Read the model definition and answer for the solid it produces. Units are mm, in the model's axes. A direction names the side the tool comes from. Give positions to 0.01 mm unless a question says otherwise; leave off trailing zeros. Order: outer loops, then holes, each group sorted by start corner. A loop starts at its lowest first (then second) coordinate and runs counter-clockwise, first axis right, second up. Notation, with made-up numbers: (35, 8) - (89, 8) arc R19 cw to (89, 44) - close; hole circle Ø11 at (-31.5, 11.25). An arc over 180 degrees is marked (long way). Write item = value, one per line.
```python
from build123d import *

# Parameters (mm, degrees)
SKETCH1_R                = 19.05
SKETCH1_R_2              = 12.7
BOSS_EXTRUDE1_DEPTH      = 571.5
BOSS_EXTRUDE2_START      = -12.7
SKETCH2_R                = 50.8
SKETCH2_R_2              = 12.7
BOSS_EXTRUDE2_DEPTH      = 12.7
SKETCH3_R                = 50.8
SKETCH3_R_2              = 12.7
BOSS_EXTRUDE3_DEPTH      = 12.7
BOSS_EXTRUDE4_REACH      = 609.748
BOSS_EXTRUDE4_END_RADIUS = 19.05
BOSS_EXTRUDE4_START      = 31.75
SKETCH4_W                = 25.4
SKETCH4_H                = 25.4
SKETCH4_R                = 2.286


with BuildPart() as part:
    # Sketch1 → Boss-Extrude1 (new, symmetric)
    with BuildSketch(Plane(origin=(0, 0, 0), x_dir=(0, 0, -1), z_dir=(1, 0, 0))):
        Circle(SKETCH1_R)
        Circle(SKETCH1_R_2, mode=Mode.SUBTRACT)
    extrude(amount=BOSS_EXTRUDE1_DEPTH, both=True)

    # Sketch2 → Boss-Extrude2 (add)
    with BuildSketch(Plane(origin=(571.5, 0, 0), x_dir=(0, 0, -1), z_dir=(1, 0, 0)).offset(BOSS_EXTRUDE2_START)):
        Circle(SKETCH2_R)
        Circle(SKETCH2_R_2, mode=Mode.SUBTRACT)
    extrude(amount=BOSS_EXTRUDE2_DEPTH)

    # Sketch3 → Boss-Extrude3 (add)
    with BuildSketch(Plane.ZY.offset(571.5)):
        with Locations(Location((0, 0, 0), (0, 0, 180))):
            Circle(SKETCH3_R)
        with Locations(Location((0, 0, 0), (0, 0, 180))):
            Circle(SKETCH3_R_2, mode=Mode.SUBTRACT)
    extrude(amount=-BOSS_EXTRUDE3_DEPTH)

    # Boss-Extrude4: up to this cylinder (the profile starts outside it)
    boss_extrude4_end = Plane(origin=(-6.170395, 0, 0), z_dir=(-1, 0, 0)) * Cylinder(BOSS_EXTRUDE4_END_RADIUS, 2008.25521, mode=Mode.PRIVATE)
    # Sketch4 → Boss-Extrude4 (add, up to the surface)
    with BuildSketch(Plane(origin=(0, 0, 0), x_dir=(1, 0, 0), z_dir=(0, 1, 0)).offset(BOSS_EXTRUDE4_START), mode=Mode.PRIVATE) as boss_extrude4_sk1:
        with Locations((-381, 0)):
            Rectangle(SKETCH4_W, SKETCH4_H)
        with Locations(Location((-381, 0, 0), (0, 0, 270))):
            Circle(SKETCH4_R, mode=Mode.SUBTRACT)
    boss_extrude4_tool1 = extrude(boss_extrude4_sk1.sketch, amount=-BOSS_EXTRUDE4_REACH, mode=Mode.PRIVATE) - boss_extrude4_end
    add(boss_extrude4_tool1.solids().sort_by_distance((-381, 31.75, 12.34079))[0])
    # Sketch4 → Boss-Extrude4 (add, up to the surface)
    with BuildSketch(Plane(origin=(0, 0, 0), x_dir=(1, 0, 0), z_dir=(0, 1, 0)).offset(BOSS_EXTRUDE4_START), mode=Mode.PRIVATE) as boss_extrude4_sk2:
        with Locations((381, 0)):
            Rectangle(SKETCH4_W, SKETCH4_H)
        with Locations(Location((381, 0, 0), (0, 0, 270))):
            Circle(SKETCH4_R, mode=Mode.SUBTRACT)
    boss_extrude4_tool2 = extrude(boss_extrude4_sk2.sketch, amount=-BOSS_EXTRUDE4_REACH, mode=Mode.PRIVATE) - boss_extrude4_end
    add(boss_extrude4_tool2.solids().sort_by_distance((368.65921, 31.75, 0))[0])


solid = part.part
```
1. For faces 4 (the face through (558.8, 1, -22)), 5 (the face through (384, 31.75, 0)), 6 (the face through (-381, 23, 12.7)), 7 (the face through (-381, 23, -12.7)), determine the directions among +Z, -Z, +X, -X, +Y, -Y from which every point of the face is accessible in a straight line to the end or side of a thin tool.
Recorded:
face_4 = none
face_5 = +Z, -Z, +Y
face_6 = +Z, +Y
face_7 = -Z, +Y
2. Flat-ended cylindrical pins translate along their axes: pin 1 (12.5 mm diameter, centred on x = -383, z = 5, fed in from +Y); pin 2 (7.5 mm diameter, centred on x = 381, z = 0, fed in from -Y); pin 3 (9 mm diameter, centred on x = 385, y = 22.5, fed in from -Z). Find the tip coordinate at first contact, or state that the pin passes through.
Recorded:
pin_1 = 31.75
pin_2 = -19.05
pin_3 = -12.7
3. Section B-B (x = 282) is taken. Determine the outline of the cut face in (y, z), and give its area (3 significant figures).
Recorded:
outline = circle Ø38.1 at (0, 0); hole circle Ø25.4 at (0, 0)
area = 633 mm^2
4. Straight lines are drawn through the part: L1, parallel to Z at x = 381, y = 26.5; L2, parallel to X at y = 17, z = -38; L3, parallel to Y at x = -75, z = 0. For each, find the intervals that lie inside material, in ascending order. Write a range as [from, to].
Recorded:
L1 = [-12.7, -2.29], [2.29, 12.7]
L2 = [-571.5, -558.8], [558.8, 571.5]
L3 = [-19.05, -12.7], [12.7, 19.05]
5. Determine the mould class of faces 1 (the face through (-8, -12.4, 2.75)), 2 (the face through (368.3, 25, 0)), 3 (the face through (7.823, -18.597, 4.13)) for opening direction Z: +Z half, -Z half, draft (parallel to the pull), parting line (faces both ways), or undercut.
Recorded:
face_1 = undercut
face_2 = draft
face_3 = parting line
6. Section A-A (y = 0) is taken. Determine the outline of the cut face in (x, z), and give its area (3 significant figures).
Recorded:
outline = (-571.5, -50.8) - (-558.8, -50.8) - (-558.8, -19.05) - (558.8, -19.05) - (558.8, -50.8) - (571.5, -50.8) - (571.5, -12.7) - (-571.5, -12.7) - close; (-571.5, 12.7) - (571.5, 12.7) - (571.5, 50.8) - (558.8, 50.8) - (558.8, 19.05) - (-558.8, 19.05) - (-558.8, 50.8) - (-571.5, 50.8) - close
area = 16,100 mm^2
